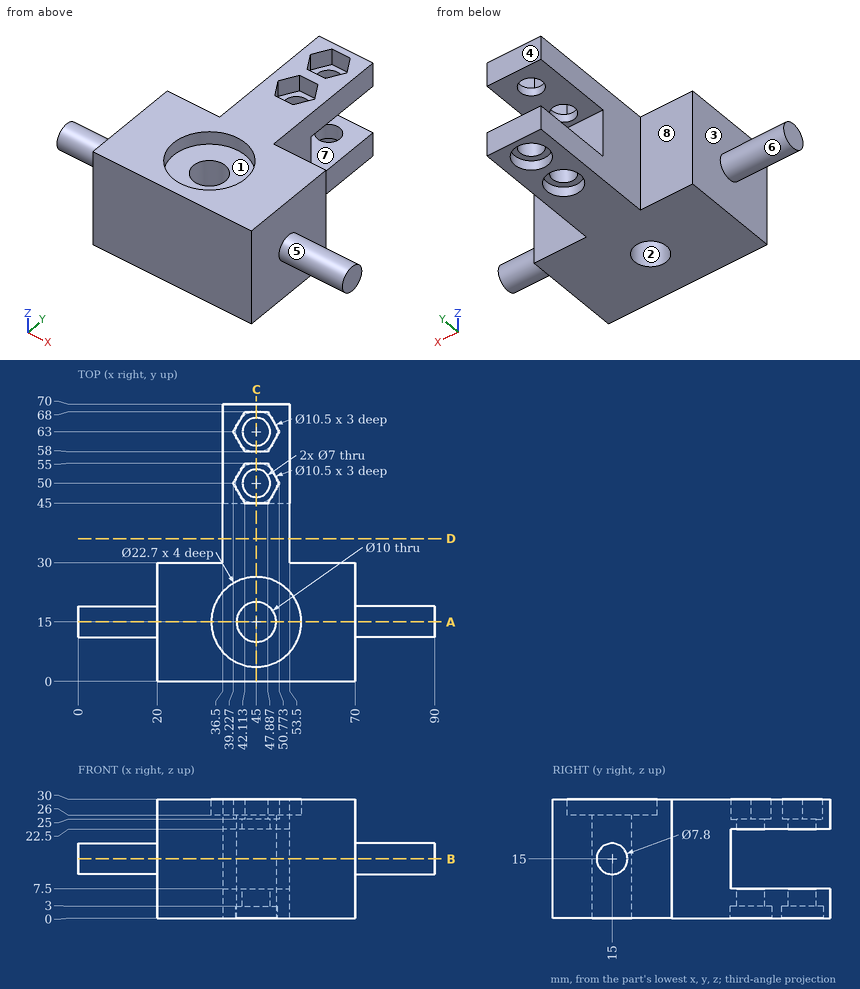
Here's the drawing with two shaded views (mm, measured from the low corner). I have some questions. A direction names the side the tool comes from. Coordinates: 2 decimals unless noted, no trailing zeros. Write each loop counter-clockwise with the first axis right and the second up, starting at its lowest first coordinate (ties: lowest second). Pieces come first, ordered by that corner, then holes. Notation, with made-up numbers: M 34.25,13 L 83.25,13 A19 cw 83.25,34 Z; hole C 10,7.25 d10. An arc over 180 degrees is marked long. Use one line per item in the form item = value.
Q1. I need wall thicknesses on line 1 along Y through (x, z) = (45, 1.8); line 2 along Y through (x, z) = (45, 23.45); line 3 along Z through (x, y) = (47.5, 56). Which ranges of each line are inside material? Lowest first, please. Write a range as from..to.
Model answer:
line_1 = 0..10, 20..44.75, 55.25..57.75, 68.25..70
line_2 = 0..10, 20..46.5, 53.5..59.5, 66.5..70
line_3 = 0..7.5, 22.5..30
Q2. If we section it at B-B (z = 15): Write out the boundary of the cut face in (x, y).
Model answer:
outline = M 0,11.1 L 20,11.1 L 20,0 L 70,0 L 70,11.1 L 90,11.1 L 90,18.9 L 70,18.9 L 70,30 L 53.5,30 L 53.5,45 L 36.5,45 L 36.5,30 L 20,30 L 20,18.9 L 0,18.9 Z; hole C 45,15 d10
Q3. If we section it at C-C (x = 45): State how many separate pieces and enclosed holes the cut face has, then the cut area to 3 significant figures.
Model answer:
separate_pieces = 6
enclosed_holes = 0
area = 1,110 mm^2
Q4. For the marked faces 5, 6, 7 and 8, which set-ups out of +Z, -Z, +X, -X, +Y, -Y let a thin tool reach every point of the face, with its end or its side?
Model answer:
face_5 = +X
face_6 = -X
face_7 = +X, -X, +Y
face_8 = +Z, -Z, -X, +Y
Q5. We'd pull the mould along Y, two halves only. Please class the marked faces 1, 2, 3 and 4: +Y half, -Y half, draft (parallel to the pull), parting line (faces both ways), or undercut.
Model answer:
face_1 = undercut
face_2 = undercut
face_3 = draft
face_4 = +Y half
Q6. If we section it at A-A (y = 15): Write out the boundary of the cut face in (x, z).
Model answer:
outline = M 0,11.1 L 20,11.1 L 20,0 L 40,0 L 40,26 L 33.65,26 L 33.65,30 L 20,30 L 20,18.9 L 0,18.9 Z; M 50,0 L 70,0 L 70,11.1 L 90,11.1 L 90,18.9 L 70,18.9 L 70,30 L 56.35,30 L 56.35,26 L 50,26 Z
Q7. For P1, Ø10, axis at y = 47, z = 22.5, coming from the +X side; P2, Ø5, axis at x = 44.5, y = 49, coming from the +Z side; P3, Ø3, axis at x = 43.5, y = 52, coming from the -Z side; P4, Ø4, axis at x = 45, y = 50, coming from the +Z side, each with a flat end and sliding along its axis, tell me the tip position at first contact or that it passes through.
Model answer:
P1 = 53.5
P2 = 25
P3 = 3
P4 = through
Q8. If we section it at D-D (y = 36): Write out the boundary of the cut face in (x, z), then the cut area to 3 significant figures.
Model answer:
outline = M 36.5,0 L 53.5,0 L 53.5,30 L 36.5,30 Z
area = 510 mm^2
